```python
from build123d import *

# Parameters (mm, degrees)
F2_R     = 3
F4_DEPTH = 20
F5_DEPTH = 20


with BuildPart() as f1:
    # F0 (on Top) → F1 (revolve)
    with BuildSketch(Plane.XY):
        with BuildLine():
            Line((-13.25, 0), (0, 0))
            Line((0, 0), (0, 37))
            Line((0, 37), (-1.5, 37))
            Line((-1.5, 37), (-1.5, 16.6235913226))
            ThreePointArc((-1.5, 16.6235913226), (-6.4401709177, 12.3947665973), (-11.3803418353, 16.6235913226))
            Line((-11.3803418353, 16.6235913226), (-11.4607692348, 17.1388115494))
            ThreePointArc((-11.4607692348, 17.1388115494), (-12.4196143352, 17.8973036522), (-13.25, 17))
            Line((-13.25, 17), (-13.25, 0))
        make_face()
    revolve(axis=Axis((0, 18.5, 0), (0, -1, 0)))

    # F2
    f2_edges = [f1.edges().sort_by_distance(p)[0] for p in [
        (1.5, 16.623591, 0),
    ]]
    fillet(f2_edges, radius=F2_R)

    # F3 (on face) → F4 (join)
    with BuildSketch(Plane.XZ):
        with BuildLine():
            Line((-12.2703911918, 5), (-38.25, 5))
            Line((-38.25, 5), (-38.25, -5))
            Line((-38.25, -5), (-12.2703911918, -5))
            ThreePointArc((-12.2703911918, -5), (-13.25, 0), (-12.2703911918, 5))
        make_face()
        with BuildLine():
            Line((12.2703911918, 5), (-12.2703911918, 5))
            ThreePointArc((-12.2703911918, 5), (-13.25, 0), (-12.2703911918, -5))
            Line((-12.2703911918, -5), (12.2703911918, -5))
            ThreePointArc((12.2703911918, -5), (13.0027916866, -2.5475298535), (13.25, 0))
            ThreePointArc((13.25, 0), (13.0027916866, 2.5475298535), (12.2703911918, 5))
        make_face()
        with BuildLine():
            Line((38.25, 5), (12.2703911918, 5))
            ThreePointArc((12.2703911918, 5), (13.0027916866, 2.5475298535), (13.25, 0))
            ThreePointArc((13.25, 0), (13.0027916866, -2.5475298535), (12.2703911918, -5))
            Line((12.2703911918, -5), (38.25, -5))
            Line((38.25, -5), (38.25, 5))
        make_face()
    extrude(amount=F4_DEPTH)

    # F5 (add): faces of the model
    f5_faces = [f1.faces().sort_by_distance(p)[0] for p in [
        (0, 0, 8.4077666552),
        (0, 0, -8.4077666552),
    ]]
    extrude(f5_faces, amount=F5_DEPTH)


solid = f1.part
```
Build history of the part. All positions in model axes, mm. A direction names the side the tool comes from. Give positions to 0.01 mm unless a question says otherwise; leave off trailing zeros. Order: outer loops, then holes, each group sorted by start corner. A loop starts at its lowest first (then second) coordinate and runs counter-clockwise, first axis right, second up. Notation, with made-up numbers: M -29,45 L 17,45 A29 ccw 17,82 Z; hole C -21.75,87.25 d4. An arc over 180 degrees is marked long. Return JSON: item names as keys, results as strings.
Q1. Flat gauge pins, fed straight in: pin 1 (10 mm diameter, centred on x = 31.5, y = -13, fed in from +Z); pin 2 (8 mm diameter, centred on x = -27.5, z = 0, fed in from +Y); pin 3 (1.5 mm diameter, centred on x = 22, z = -6.5, fed in from -Y); pin 4 (16 mm diameter, centred on x = 21, y = -8, fed in from -Z). Where does each tip first touch, or does it go through?
Answer list:
{"pin 1": "stops at z = 5", "pin 2": "stops at y = 0", "pin 3": "passes through", "pin 4": "stops at z = -5"}
Q2. Band-saw the part on C-C (y = 3). Give the cut face in (x, z), then the cut area to 3 significant figures.
Answer list:
{"outline": "C 0,0 d26.5", "area": "552 mm^2"}
Q3. Band-saw the part on A-A (y = -7). Give the cut face in (x, z).
Answer list:
{"outline": "M -38.25,-5 L -12.27,-5 A13.25 ccw 12.27,-5 L 38.25,-5 L 38.25,5 L 12.27,5 A13.25 ccw -12.27,5 L -38.25,5 Z"}
Q4. Wall check: probe 1 along Z at (x, y) = (30, -3); probe 2 along X at (y, z) = (23, 0); probe 3 along Y at (x, z) = (-14.5, 1). Give the ranges that are in metal, low to high. Write a range as from..to.
Answer list:
{"probe 1": "z = -5..5", "probe 2": "x = -1.5..1.5", "probe 3": "y = -20..0"}
Q5. 3-axis set-ups, long thin cutter, end or side, ignore diameter. For faces 1 (the face through (25, -10, -5)), 2 (the face through (-25, -10, 5)), 3 (the face through (-25, -10, -5)), 4 (the face through (25, -10, 5)), 5 (the face through (-1.43, 26.81, -0.45)): which of +Z, -Z, +X, -X, +Y, -Y reach the whole face in a straight line?
Answer list:
{"face 1": "-Z, +X, +Y, -Y", "face 2": "+Z, -X, +Y, -Y", "face 3": "-Z, -X, +Y, -Y", "face 4": "+Z, +X, +Y, -Y", "face 5": "+Y"}
Q6. Band-saw the part on D-D (y = 20.5). Give the cut face in (x, z), then the cut area to 3 significant figures.
Answer list:
{"outline": "C 0,0 d3", "area": "7.07 mm^2"}
Q7. Band-saw the part on B-B (x = -18). Give the cut face in (y, z), then the cut area to 3 significant figures.
Answer list:
{"outline": "M -20,-5 L 0,-5 L 0,5 L -20,5 Z", "area": "200 mm^2"}
